Work out the finished part from the listing and answer in its coordinate system (mm). Face numbers are marked on the shaded views. A direction names the side the tool comes from. Round coordinates to 2 decimals unless told otherwise and drop trailing zeros. Order: outer loops, then holes, each group sorted by start corner. A loop starts at its lowest first (then second) coordinate and runs counter-clockwise, first axis right, second up.
from build123d import *

# Parameters (mm, degrees)
F1_R      = 4.1
F2_DEPTH  = 40
F3_R      = 11
F4_DEPTH  = 17
F5_W      = 6
F5_H      = 3
F6_DEPTH  = 60
F7_R      = 1.6
F8_DEPTH  = 19
F10_DEPTH = 17
F11_W     = 2
F11_H     = 7
F11_H_2   = 2
F11_W_2   = 26
F12_DEPTH = 15
F13_R     = 1.6
F14_DEPTH = 17
F16_DEPTH = 4.5
F19_DEPTH = 15
F21_R     = 1.6
F22_DEPTH = 10
F24_DEPTH = 46.5


# Not quite as in the source:
# - a pattern or mirror of a feature is missing from the dataset's text; its kind, count and spacing are read off the source's solid


with BuildPart() as f2:
    # F1 (on Right) → F2 (new body)
    with BuildSketch(Plane.YZ):
        with BuildLine():
            ThreePointArc((-35, 8.5), (-32.5104076401, 2.4895923599), (-26.5, 0))
            Line((-26.5, 0), (26.5, 0))
            ThreePointArc((26.5, 0), (32.5104076401, 2.4895923599), (35, 8.5))
            ThreePointArc((35, 8.5), (32.5104076401, 14.5104076401), (26.5, 17))
            Line((26.5, 17), (-26.5, 17))
            ThreePointArc((-26.5, 17), (-32.5104076401, 14.5104076401), (-35, 8.5))
        make_face()
        with Locations((-25, 8.5)):
            Circle(F1_R, mode=Mode.SUBTRACT)
        with Locations((25, 8.5)):
            Circle(F1_R, mode=Mode.SUBTRACT)
    extrude(amount=-F2_DEPTH)

    # F3 (on Top) → F4 (cut)
    with BuildSketch(Plane.XY):
        Circle(F3_R)
    extrude(amount=F4_DEPTH, mode=Mode.SUBTRACT)

    # F5 (on Top) → F6 (join)
    with BuildSketch(Plane.XY):
        with BuildLine():
            Line((9.5, 6.5), (9.5, 9.5))
            Line((9.5, 9.5), (-1.5, 9.5))
            ThreePointArc((-1.5, 9.5), (-7.1568542495, 7.1568542495), (-9.5, 1.5))
            Line((-9.5, 1.5), (-9.5, -1.5))
            ThreePointArc((-9.5, -1.5), (-7.1568542495, -7.1568542495), (-1.5, -9.5))
            Line((-1.5, -9.5), (9.5, -9.5))
            Line((9.5, -9.5), (9.5, -6.5))
            Line((9.5, -6.5), (2.8565713714, -6.5))
            ThreePointArc((2.8565713714, -6.5), (-7.1, 0), (2.8565713714, 6.5))
            Line((2.8565713714, 6.5), (9.5, 6.5))
        make_face()
        with Locations((-12.5, 0)):
            Rectangle(F5_W, F5_H)
    extrude(amount=F6_DEPTH)

    # F7 (on face) → F8 (cut)
    with BuildSketch(Plane.XZ.offset(9.5)):
        with Locations((6.5, 50)):
            Circle(F7_R)
        with Locations((6.5, 10)):
            Circle(F7_R)
    extrude(amount=-F8_DEPTH, mode=Mode.SUBTRACT)

    # F9 (on Top) → F10 (cut)
    with BuildSketch(Plane.XY):
        with BuildLine():
            ThreePointArc((-19, 0), (-22.2218254069, 7.7781745931), (-30, 11))
            Line((-30, 11), (-41, 11))
            Line((-41, 11), (-41, -11))
            Line((-41, -11), (-30, -11))
            ThreePointArc((-30, -11), (-22.2218254069, -7.7781745931), (-19, 0))
        make_face()
    extrude(amount=F10_DEPTH, mode=Mode.SUBTRACT)

    # F11 (on offset) → F12 (cut)
    with BuildSketch(Plane.XZ.offset(21)):
        with Locations((-6, 3.5)):
            Rectangle(F11_W, F11_H)
        with Locations((-6, 8)):
            Rectangle(F11_W, F11_H_2)
        with Locations((-20, 8)):
            Rectangle(F11_W_2, F11_H_2)
        with Locations((-34, 8)):
            Rectangle(F11_W, F11_H_2)
        with Locations((-34, 3.5)):
            Rectangle(F11_W, F11_H)
    f12 = extrude(amount=F12_DEPTH, mode=Mode.SUBTRACT)

    # F12_copies: F12 across plane
    add(f12.mirror(Plane.ZX), mode=Mode.SUBTRACT)

    # F13 (on Top) → F14 (cut)
    with BuildSketch(Plane.XY):
        with Locations((-20, -31.8666002653)):
            Circle(F13_R)
    f14 = extrude(amount=F14_DEPTH, mode=Mode.SUBTRACT)

    # F14_copies: F14 across plane
    add(f14.mirror(Plane.ZX), mode=Mode.SUBTRACT)

    # F15 (on face) → F16 (cut)
    with BuildSketch(Plane.XY.offset(17)):
        Polygon((-21.6165807537, -29.0666002653), (-23.2331615075, -31.8666002653), (-21.6165807537, -34.6666002653), (-18.3834192463, -34.6666002653), (-16.7668384925, -31.8666002653), (-18.3834192463, -29.0666002653), align=None)
    f16 = extrude(amount=-F16_DEPTH, mode=Mode.SUBTRACT)

    # F16_copies: F16 across plane
    add(f16.mirror(Plane.ZX), mode=Mode.SUBTRACT)

    # F18 (on face) → F19 (join)
    with BuildSketch(Plane(origin=(-40, 0, 0), x_dir=(0, -1, 0), z_dir=(-1, 0, 0))):
        Polygon((34.8862050714, 9.8862050714), (45, 20), (35, 20), (29.8862050714, 14.8862050714), align=None)
    f19 = extrude(amount=-F19_DEPTH)

    # F19_copies: F19 across plane
    add(f19.mirror(Plane(origin=(-20, 0, 0), x_dir=(0, 0, 1), z_dir=(1, 0, 0))))

    # F21 (on offset) → F22 (join)
    with BuildSketch(Plane.XZ.offset(45)):
        Polygon((-40, 20), (0, 20), (0, 60), (-10, 60), (-20, 60), (-20, 55), (-10, 45), (-10, 30), (-40, 30), align=None)
        with Locations((-35, 25)):
            Circle(F21_R, mode=Mode.SUBTRACT)
        with Locations((-5, 25)):
            Circle(F21_R, mode=Mode.SUBTRACT)
        with Locations((-5, 55)):
            Circle(F21_R, mode=Mode.SUBTRACT)
    extrude(amount=-F22_DEPTH)

    # F23 (on face) → F24 (join)
    with BuildSketch(Plane(origin=(0, 1.5, 0), x_dir=(-1, 0, 0), z_dir=(0, 1, 0))):
        Polygon((20, 60), (10, 60), (10, 50), (15, 50), (20, 55), align=None)
    extrude(amount=-F24_DEPTH)


solid = f2.part
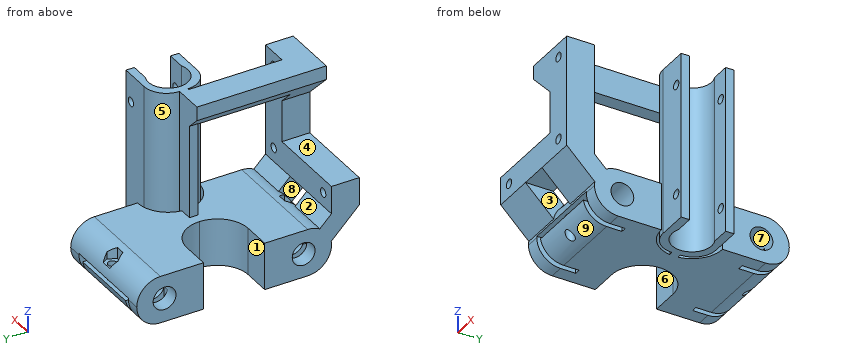
Item 1: Find section C-C (y = -12). Write down the section's boundary in (x, z).
Item 2: Find section B-B (z = 25). Write down the section's boundary in (x, y), plus the area to 3 significant figures.
Item 3: For a pull along Y with two mould halves and no side action, classify the marked faces 6, 7, 8 and 9 as released by +Y, released by -Y, zero draft, split by the parting line, or undercut.
Item 4: A tool of negligible diameter and unlimited length cuts with its end or side. For the marked faces 1, 2, 3, 4 and 5, from which of +Z, -Z, +X, -X, +Y, -Y can it reach the whole face along a straight path? Write none if from no direction.
Item 5: Find section D-D (y = 25). Write down the section's boundary in (x, z).
Item 6: Find the intervals of material crossed by line 1 along Z through (x, y) = (6.5, -8.8); line 2 along Z through (x, y) = (-5, -37.5); line 3 along Z through (x, y) = (-15, -6), in increasing order.
Item 7: Find section A-A (x = 6.5). Write down the section's boundary in (y, z), plus the area to 3 significant figures.
Item 8: Given pin 1 (10 mm diameter, centred on y = 29.5, z = 5.5, fed in from +X); pin 2 (4.5 mm diameter, centred on x = -13.5, y = 31, fed in from -Z); pin 3 (5.5 mm diameter, centred on y = -12, z = 58.5, fed in from -X); pin 4 (10 mm diameter, centred on y = -26, z = 6.5, fed in from -X), each flat-ended and moving along its own axis, determine where each tip first touches the part or whether it passes through.
Model answer:
1. outline: (-40, 0) - (0, 0) - (0, 17) - (-40, 17) - close; (-20, 55) - (-15, 50) - (-10, 50) - (-10, 60) - (-20, 60) - close
2. outline: (-40, -45) - (-36.6, -45) - (-36.6, -35) - (-40, -35) - close; (-33.4, -45) - (-6.6, -45) - (-6.6, -35) - (-33.4, -35) - close; (-15.5, -1.5) - (-9.5, -1.5) arc R8 ccw to (-1.5, -9.5) - (9.5, -9.5) - (9.5, -6.5) - (2.86, -6.5) arc R7.1 cw (long way) to (2.86, 6.5) - (9.5, 6.5) - (9.5, 9.5) - (-1.5, 9.5) arc R8 ccw to (-9.5, 1.5) - (-15.5, 1.5) - close; (-3.4, -45) - (0, -45) - (0, -35) - (-3.4, -35) - close
2. area: 483 mm2
3. face 6: undercut
3. face 7: undercut
3. face 8: zero draft
3. face 9: released by -Y
4. face 1: +Z, -Z, -X
4. face 2: +Z, +X, -X
4. face 3: -Y
4. face 4: -X, -Y
4. face 5: +Z, -Z
5. outline: (-40, 0) - (-35, 0) - (-35, 4.4) - (-40, 4.4) - close; (-40, 12.6) - (0, 12.6) - (0, 17) - (-40, 17) - close; (-33, 0) - (-7, 0) - (-7, 4.4) - (-33, 4.4) - close; (-5, 0) - (0, 0) - (0, 4.4) - (-5, 4.4) - close
6. line 1: z = 0 to 8.4, 11.6 to 48.4, 51.6 to 60
6. line 2: z = 12.5 to 23.4, 26.6 to 53.4, 56.6 to 60
6. line 3: z = 0 to 17, 50 to 60
7. outline: (-9.5, 0) - (-6.5, 0) - (-6.5, 8.4) - (-9.5, 8.4) - close; (-9.5, 11.6) - (-6.5, 11.6) - (-6.5, 48.4) - (-9.5, 48.4) - close; (-9.5, 51.6) - (-6.5, 51.6) - (-6.5, 60) - (-9.5, 60) - close; (6.5, 0) - (9.5, 0) - (9.5, 8.4) - (6.5, 8.4) - close; (6.5, 11.6) - (9.5, 11.6) - (9.5, 48.4) - (6.5, 48.4) - close; (6.5, 51.6) - (9.5, 51.6) - (9.5, 60) - (6.5, 60) - close
7. area: 322 mm2
8. pin 1: stops at x = 0
8. pin 2: stops at z = 0.3
8. pin 3: stops at x = -20
8. pin 4: stops at x = -40
